```python
from build123d import *

# Parameters (mm, degrees)
SKETCH1_W           = 8.4
SKETCH1_H           = 22.5
BOSS_EXTRUDE1_DEPTH = 1
SKETCH2_R           = 1
BOSS_EXTRUDE2_DEPTH = 1
BOSS_EXTRUDE3_START = -21.5
SKETCH2_2_R         = 1
BOSS_EXTRUDE3_DEPTH = 1
SKETCH1_3_W         = 11.6
SKETCH1_3_H         = 22.5
BOSS_EXTRUDE4_DEPTH = 1
BOSS_EXTRUDE5_DEPTH = 8.4
FILLET2_R           = 1
SKETCH4_R           = 0.902238409
CUT_EXTRUDE1_DEPTH  = 23.614375959


with BuildPart() as part:
    # Sketch1 → Boss-Extrude1 (new body)
    with BuildSketch(Plane.XY):
        Rectangle(SKETCH1_W, SKETCH1_H)
    extrude(amount=BOSS_EXTRUDE1_DEPTH)

    # Sketch2 → Boss-Extrude2 (add)
    with BuildSketch(Plane(origin=(0, 11.25, 0), x_dir=(1, 0, 0), z_dir=(0, 1, 0))):
        with BuildLine():
            Line((-2, -12), (-4.2, -1))
            Line((-4.2, -1), (4.2, -1))
            Line((4.2, -1), (2, -12))
            ThreePointArc((2, -12), (0, -14), (-2, -12))
        make_face()
        with Locations(Location((0, -12, 0), (0, 0, 270))):
            Circle(SKETCH2_R, mode=Mode.SUBTRACT)
    extrude(amount=-BOSS_EXTRUDE2_DEPTH)

    # Sketch2<2> → Boss-Extrude3 (add)
    with BuildSketch(Plane(origin=(0, 11.25, 0), x_dir=(1, 0, 0), z_dir=(0, 1, 0)).offset(BOSS_EXTRUDE3_START)):
        with BuildLine():
            Line((-2, -12), (-4.2, -1))
            Line((-4.2, -1), (4.2, -1))
            Line((4.2, -1), (2, -12))
            ThreePointArc((2, -12), (0, -14), (-2, -12))
        make_face()
        with Locations(Location((0, -12, 0), (0, 0, 270))):
            Circle(SKETCH2_2_R, mode=Mode.SUBTRACT)
    extrude(amount=-BOSS_EXTRUDE3_DEPTH)

    # Sketch1<3> → Boss-Extrude4 (add)
    with BuildSketch(Plane.XY):
        with Locations((-10, 0)):
            Rectangle(SKETCH1_3_W, SKETCH1_3_H)
    extrude(amount=BOSS_EXTRUDE4_DEPTH)

    # Sketch3 → Boss-Extrude5 (add)
    with BuildSketch(Plane(origin=(0, 0, 0), x_dir=(-1, 0, 0), z_dir=(0, 0, -1))):
        Polygon((2.3, 8.1), (7.2, 8.1), (7.2, 11.1), (7.8, 11.1), (7.8, 8.1), (11.8, 8.1), (11.8, 9.1), (8.8, 9.1), (8.8, 12.1), (6.2, 12.1), (6.2, 9.1), (2.3, 9.1), align=None)
    extrude(amount=BOSS_EXTRUDE5_DEPTH)

    # Fillet2
    # the kernel refuses this fillet: 1 mm, written as the material it adds along each edge
    with BuildSketch(Plane(origin=(-6.2, 11.25, 0), x_dir=(1, 0, 0), z_dir=(0, -1, 0))) as fillet2_piece_1_section:
        with BuildLine():
            CenterArc((FILLET2_R, -FILLET2_R), FILLET2_R, 90, 90)
            Line((0, -FILLET2_R), (0, 0))
            Line((0, 0), (FILLET2_R, 0))
        make_face()
    fillet2_piece_1 = extrude(amount=4.65, mode=Mode.PRIVATE)
    fillet2_piece_1 = split(fillet2_piece_1, bisect_by=Plane(origin=(-6.2, 8.1, 0), z_dir=(0, 1, 0)), keep=Keep.TOP, mode=Mode.PRIVATE)
    add(fillet2_piece_1)
    with BuildSketch(Plane(origin=(-8.8, 9.1, 0), x_dir=(-1, 0, 0), z_dir=(0, 1, 0))) as fillet2_piece_2:
        with BuildLine():
            CenterArc((FILLET2_R, -FILLET2_R), FILLET2_R, 90, 90)
            Line((0, -FILLET2_R), (0, 0))
            Line((0, 0), (FILLET2_R, 0))
        make_face()
    extrude(amount=2.15)
    with BuildSketch(Plane(origin=(-8.8, 9.1, 2.5), x_dir=(-1, 0, 0), z_dir=(0, 0, -1))) as fillet2_piece_3_section:
        with BuildLine():
            CenterArc((FILLET2_R, FILLET2_R), FILLET2_R, 180, 90)
            Line((0, FILLET2_R), (0, 0))
            Line((0, 0), (FILLET2_R, 0))
        make_face()
    fillet2_piece_3 = extrude(amount=10.9, mode=Mode.PRIVATE)
    fillet2_piece_3 = split(fillet2_piece_3, bisect_by=Plane(origin=(-8.8, 9.1, 1), z_dir=(0, 0, -1)), keep=Keep.TOP, mode=Mode.PRIVATE)
    add(fillet2_piece_3)
    with BuildSketch(Plane(origin=(-6.2, 9.1, 2.5), x_dir=(0, 1, 0), z_dir=(0, 0, -1))) as fillet2_piece_4_section:
        with BuildLine():
            CenterArc((FILLET2_R, FILLET2_R), FILLET2_R, 180, 90)
            Line((0, FILLET2_R), (0, 0))
            Line((0, 0), (FILLET2_R, 0))
        make_face()
    fillet2_piece_4 = extrude(amount=10.9, mode=Mode.PRIVATE)
    fillet2_piece_4 = split(fillet2_piece_4, bisect_by=Plane(origin=(-6.2, 9.1, 1), z_dir=(0, 0, -1)), keep=Keep.TOP, mode=Mode.PRIVATE)
    add(fillet2_piece_4)
    # the kernel refuses this fillet: 1 mm, written as the material it takes off along each edge
    with BuildSketch(Plane(origin=(-2.3, 9.1, 0), x_dir=(-1, 0, 0), z_dir=(0, 0, -1)), Plane(origin=(-11.8, 9.1, 0), x_dir=(0, -1, 0), z_dir=(0, 0, -1))) as fillet2_2_piece_1:
        with BuildLine():
            CenterArc((FILLET2_R, -FILLET2_R), FILLET2_R, 90, 90)
            Line((0, -FILLET2_R), (0, 0))
            Line((0, 0), (FILLET2_R, 0))
        make_face()
    extrude(amount=10.9, mode=Mode.SUBTRACT)
    with BuildSketch(Plane(origin=(-11.271714992, 12.1, 0), x_dir=(0, 0, -1), z_dir=(1, 0, 0))) as fillet2_2_piece_2:
        with BuildLine():
            CenterArc((0.988685997, -1), FILLET2_R, 90, 81.373073441)
            Line((0, -0.85), (0, 0))
            Line((0, 0), (0.988685997, 0))
        make_face()
    extrude(amount=7.543429983, mode=Mode.SUBTRACT)
    # the kernel refuses this fillet: 1 mm, written as the material it adds along each edge
    with BuildSketch(Plane(origin=(-5.2, 10.1, -1), x_dir=(0, -1, 0), z_dir=(0, 0, 1))) as fillet2_3_piece_1_section:
        Polygon((0, 0), (FILLET2_R * 1.02, 0), (FILLET2_R * 1.02, -FILLET2_R * 1.02), (0, -FILLET2_R * 1.02), align=None)
    fillet2_3_piece_1 = extrude(amount=FILLET2_R * 1.02, mode=Mode.PRIVATE)
    fillet2_3_piece_1 = fillet2_3_piece_1 - Plane(origin=(-5.2, 10.1, -1), x_dir=(0.7071067811865475, 0.7071067811865475, 0), z_dir=(0, 0, 1)) * Sphere(FILLET2_R, mode=Mode.PRIVATE)
    add(fillet2_3_piece_1)
    with BuildSketch(Plane(origin=(-9.8, 10.1, -1), x_dir=(0, -1, 0), z_dir=(0, 0, 1))) as fillet2_3_piece_2_section:
        Polygon((0, 0), (FILLET2_R * 1.02, 0), (FILLET2_R * 1.02, FILLET2_R * 1.02), (0, FILLET2_R * 1.02), align=None)
    fillet2_3_piece_2 = extrude(amount=FILLET2_R * 1.02, mode=Mode.PRIVATE)
    fillet2_3_piece_2 = fillet2_3_piece_2 - Plane(origin=(-9.8, 10.1, -1), x_dir=(-0.7071067811865475, 0.7071067811865475, 0), z_dir=(0, 0, 1)) * Sphere(FILLET2_R, mode=Mode.PRIVATE)
    add(fillet2_3_piece_2)
    with BuildSketch(Plane(origin=(-10.8, 9.1, 0), x_dir=(0, 1, 0), z_dir=(1, 0, 0))) as fillet2_3_piece_3:
        with BuildLine():
            CenterArc((FILLET2_R, -FILLET2_R), FILLET2_R, 90, 90)
            Line((0, -FILLET2_R), (0, 0))
            Line((0, 0), (FILLET2_R, 0))
        make_face()
    extrude(amount=1)
    with BuildSketch(Plane(origin=(-5.2, 9.1, 0), x_dir=(0, 1, 0), z_dir=(1, 0, 0))) as fillet2_3_piece_4:
        with BuildLine():
            CenterArc((FILLET2_R, -FILLET2_R), FILLET2_R, 90, 90)
            Line((0, -FILLET2_R), (0, 0))
            Line((0, 0), (FILLET2_R, 0))
        make_face()
    extrude(amount=1.9)
    with BuildSketch(Plane(origin=(-3.3, 8.1, 0), x_dir=(0, 1, 0), z_dir=(-1, 0, 0))) as fillet2_3_piece_5:
        with BuildLine():
            CenterArc((1 + FILLET2_R, FILLET2_R), FILLET2_R, 180, 90)
            Line((1, FILLET2_R), (1, 0))
            Line((1, 0), (1 + FILLET2_R, 0))
        make_face()
    revolve(axis=Axis((-3.3, 8.1, 0), (0, 0, -1)), revolution_arc=90)
    with BuildSketch(Plane(origin=(-10.8, 8.1, 0), x_dir=(-1, 0, 0), z_dir=(0, -1, 0))) as fillet2_3_piece_6:
        with BuildLine():
            CenterArc((1 + FILLET2_R, FILLET2_R), FILLET2_R, 180, 90)
            Line((1, FILLET2_R), (1, 0))
            Line((1, 0), (1 + FILLET2_R, 0))
        make_face()
    revolve(axis=Axis((-10.8, 8.1, 0), (0, 0, -1)), revolution_arc=90)

    # Sketch4 → Cut-Extrude1 (cut, symmetric)
    with BuildSketch(Plane.ZY.offset(8.8)):
        with Locations(Location((-4.2, 9.6, 0), (0, 0, 33.654064464))):
            Circle(SKETCH4_R)
    extrude(amount=CUT_EXTRUDE1_DEPTH, both=True, mode=Mode.SUBTRACT)

    # Mirror1: read off the stored shape, not the designer's step
    # Mirror1: part across plane


with BuildPart() as part_1:
    add(part.part)
    add(part.part.mirror(Plane.ZX))


solid = part_1.part
```
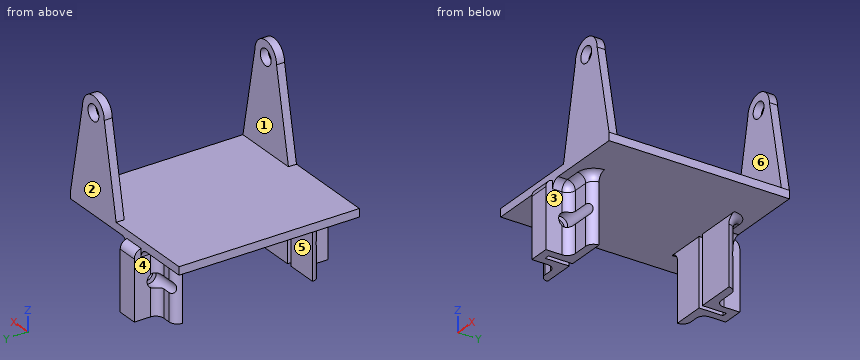
The model under review builds one solid part; all positions refer to its coordinate system, in mm. Face numbers are marked on the shaded views. A direction names the side the tool comes from. Coordinates: 2 decimals unless noted, no trailing zeros. Write each loop counter-clockwise with the first axis right and the second up, starting at its lowest first coordinate (ties: lowest second). Pieces come first, ordered by that corner, then holes. Notation, with made-up numbers: (66.5, 22) -> (90.5, 22) arc R22 ccw to (90.5, 59) -> close; hole circle Ø7 at (78, -9.5). An arc over 180 degrees is marked (long way). One line per item, written item: value. Start each with the question number.
Q1. Add section C-C, the plane z = 2.75. Give the boundary of the cut face in (x, y).
Q2. To check wall thickness, follow probe 1 along Y at (x, z) = (-9.75, -4.2); probe 2 along X at (y, z) = (10.55, 12); probe 3 along Y at (x, z) = (-6.75, -4). State the ranges of each line that lie inside material, in increasing order.
Q3. Add section B-B, the plane x = 0. Give the boundary of the cut face in (y, z).
Q4. Clearance check with flat-ended pins moving along their axes: P1, Ø6.5, axis at x = 1, z = 10, coming from the +Y side; P2, Ø5, axis at x = -12, y = 7, coming from the +Z side; P3, Ø4, axis at y = -9, z = 11.5, coming from the -X side. State where each tip first meets the part, or that it passes through.
Q5. Add section D-D, the plane y = -6. Give the boundary of the cut face in (x, z).
Q6. For the marked faces 4, 5 and 6, list the 3-axis set-ups (+Z, -Z, +X, -X, +Y, -Y) from which the entire face can be reached by the end or side of a thin tool; tool diameter is ignored.
Q7. The part is to be moulded in two halves that separate along Y. For the marked faces 1, 2 and 3, say which applies: +Y half, -Y half, draft (parallel to the pull), parting line (faces both ways), or undercut.
Q8. Add section A-A, the plane z = -2.5. Give the boundary of the cut face in (x, y).
Response:
1. outline: (-3.85, -11.25) -> (3.85, -11.25) -> (3.85, -10.25) -> (-3.85, -10.25) -> close; (-3.85, 10.25) -> (3.85, 10.25) -> (3.85, 11.25) -> (-3.85, 11.25) -> close
2. probe 1: -8.7 to -8.1, 8.1 to 8.7
2. probe 2: -2 to -1, 1 to 2
2. probe 3: -12.1 to -10.48, -8.72 to -8.1, 8.1 to 8.72, 10.48 to 12.1
3. outline: (-11.25, 0) -> (11.25, 0) -> (11.25, 11) -> (10.25, 11) -> (10.25, 1) -> (-10.25, 1) -> (-10.25, 11) -> (-11.25, 11) -> close; (-11.25, 13) -> (-10.25, 13) -> (-10.25, 14) -> (-11.25, 14) -> close; (10.25, 13) -> (11.25, 13) -> (11.25, 14) -> (10.25, 14) -> close
4. P1: y = 11.25
4. P2: z = 1
4. P3: x = -2.41
5. outline: (-15.8, 0) -> (4.2, 0) -> (4.2, 1) -> (-15.8, 1) -> close
6. face 4: -Z, -X, +Y
6. face 5: -Z, +X, -X
6. face 6: +Z, +X, -X
7. face 1: undercut
7. face 2: +Y half
7. face 3: draft
8. outline: (-11.8, -8.1) arc R1 ccw to (-10.8, -9.1) -> (-9.8, -9.1) arc R1 cw to (-8.8, -10.1) -> (-8.8, -12.1) -> (-6.2, -12.1) -> (-6.2, -10.1) arc R1 cw to (-5.2, -9.1) -> (-3.3, -9.1) arc R1 ccw to (-2.3, -8.1) -> (-7.2, -8.1) -> (-7.2, -11.1) -> (-7.8, -11.1) -> (-7.8, -8.1) -> close; (-11.8, 8.1) -> (-7.8, 8.1) -> (-7.8, 11.1) -> (-7.2, 11.1) -> (-7.2, 8.1) -> (-2.3, 8.1) arc R1 ccw to (-3.3, 9.1) -> (-5.2, 9.1) arc R1 cw to (-6.2, 10.1) -> (-6.2, 12.1) -> (-8.8, 12.1) -> (-8.8, 10.1) arc R1 cw to (-9.8, 9.1) -> (-10.8, 9.1) arc R1 ccw to start
